Geometry: see drawing. Coordinates: mm, zero at the bounding-box minimum. Give positions to 0.01 mm unless a question says otherwise; leave off trailing zeros. Write each loop counter-clockwise with the first axis right and the second up, starting at its lowest first coordinate (ties: lowest second). Pieces come first, ordered by that corner, then holes. Notation, with made-up numbers: (30.25, 65.25) -> (53.25, 65.25) arc R25 ccw to (53.25, 103.25) -> close; hole circle Ø5 at (31, 14). An arc over 180 degrees is marked (long way). Use one line per item in the form item = value. Start each with the question number.
(1) Cut plane A-A, the plane y = 1.2. Output: boundary loops of the cut face in (x, z) (1 decimal).
(2) Draft query along X for the marked faces 1 and 2. Return one class per face: pulls with the +X half, pulls with the -X half, needs draft (parallel to the pull), parting line crosses it, or undercut.
(3) Cut plane C-C, the plane z = 15.25. Output: boundary loops of the cut face in (x, y).
(4) Material intervals for line 1 along X through (y, z) = (1.8, 8.5) (1 decimal); line 2 along Z through (x, y) = (5.75, 0.35); line 3 along X through (y, z) = (0.75, 16.75), sorted ascending. Write a range as from..to.
(5) First-contact query: P1, Ø0.6, axis at y = 1.5, z = 14, coming from the -X side. Flat tip, straight axial feed; report the tip coordinate or a pass-through.
(6) Cut plane B-B, the plane x = 5.5. Output: boundary loops of the cut face in (y, z), and give its area (3 significant figures).
(7) Cut plane D-D, the plane x = 2.5. Output: boundary loops of the cut face in (y, z).
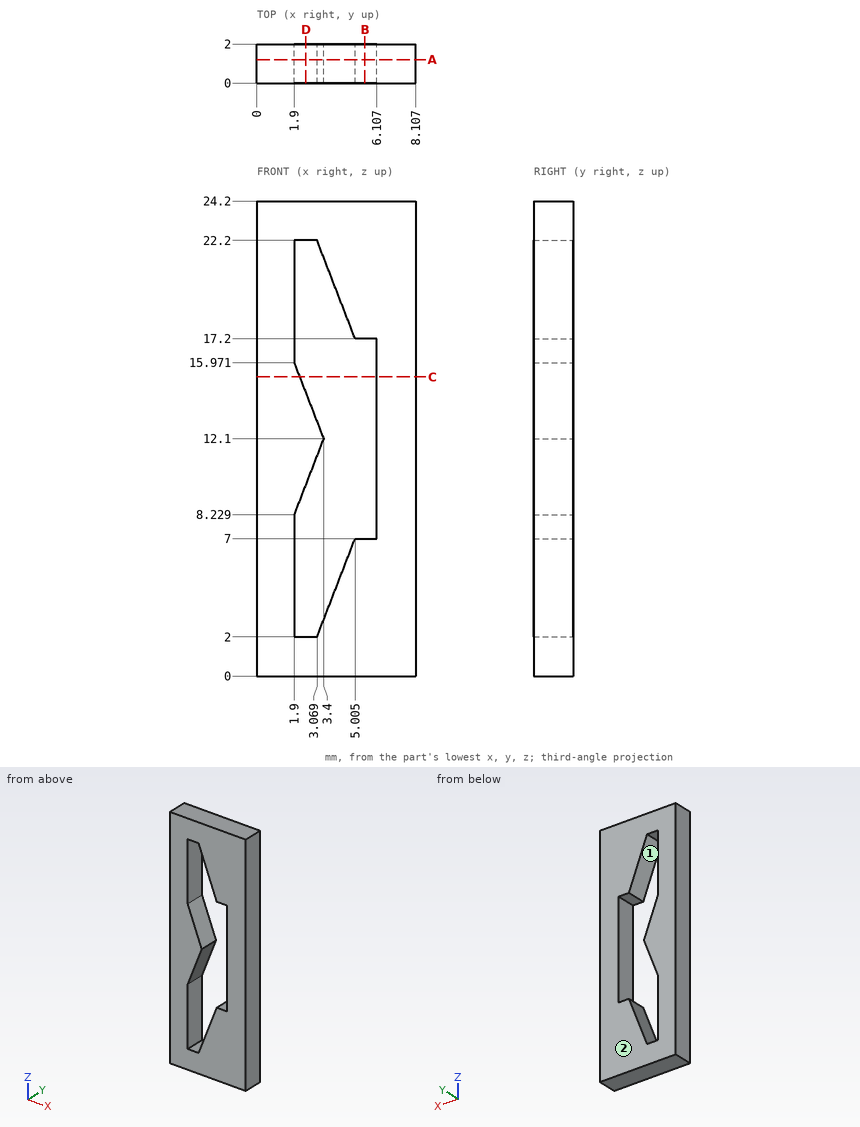
Geometry says:
q1.outline = (0, 0) -> (8.1, 0) -> (8.1, 24.2) -> (0, 24.2) -> close; hole (1.9, 2) -> (3.1, 2) -> (5, 7) -> (6.1, 7) -> (6.1, 17.2) -> (5, 17.2) -> (3.1, 22.2) -> (1.9, 22.2) -> (1.9, 16) -> (3.4, 12.1) -> (1.9, 8.2) -> close
q2.face_1 = undercut
q2.face_2 = needs draft
q3.outline = (0, 0) -> (2.18, 0) -> (2.18, 2) -> (0, 2) -> close; (6.11, 0) -> (8.11, 0) -> (8.11, 2) -> (6.11, 2) -> close
q4.line_1 = 0..2, 6.1..8.1
q4.line_2 = 0..7, 17.2..24.2
q4.line_3 = 0..1.9, 6.11..8.11
q5.P1 = 0
q6.outline = (0, 0) -> (2, 0) -> (2, 7) -> (0, 7) -> close; (0, 17.2) -> (2, 17.2) -> (2, 24.2) -> (0, 24.2) -> close
q6.area = 28.0 mm^2
q7.outline = (0, 0) -> (2, 0) -> (2, 2) -> (0, 2) -> close; (0, 9.78) -> (2, 9.78) -> (2, 14.42) -> (0, 14.42) -> close; (0, 22.2) -> (2, 22.2) -> (2, 24.2) -> (0, 24.2) -> close
